```python
from build123d import *

# Parameters (mm, degrees)
SKETCH1_W           = 29
SKETCH1_H           = 39
BOSS_EXTRUDE1_DEPTH = 40
SKETCH2_R           = 10.1
BOSS_EXTRUDE2_DEPTH = 33
SKETCH3_R           = 20
BOSS_EXTRUDE3_DEPTH = 2.5
FILLET1_R           = 5


with BuildPart() as part:
    # Sketch1 → Boss-Extrude1 (new body)
    with BuildSketch(Plane(origin=(0, 0, 0), x_dir=(1, 0, 0), z_dir=(0, 1, 0))):
        Rectangle(SKETCH1_W, SKETCH1_H)
    extrude(amount=BOSS_EXTRUDE1_DEPTH)

    # Sketch2 → Boss-Extrude2 (add)
    with BuildSketch(Plane(origin=(0, 40, 0), x_dir=(1, 0, 0), z_dir=(0, 1, 0))):
        with Locations(Location((0, 0, 0), (0, 0, 270))):
            Circle(SKETCH2_R)
    extrude(amount=BOSS_EXTRUDE2_DEPTH)

    # Sketch3 → Boss-Extrude3 (add)
    with BuildSketch(Plane(origin=(0, 73, 0), x_dir=(1, 0, 0), z_dir=(0, 1, 0))):
        with Locations(Location((0, 0, 0), (0, 0, 270))):
            Circle(SKETCH3_R)
    extrude(amount=-BOSS_EXTRUDE3_DEPTH)

    # Fillet1
    # the kernel refuses this fillet: 5 mm, written as the material it takes off along each edge
    with BuildSketch(Plane(origin=(0, 73, 0), x_dir=(0, 0, 1), z_dir=(-1, 0, 0))) as fillet1_piece_1:
        with BuildLine():
            CenterArc((15.669872981, -5), FILLET1_R, 30, 60)
            Line((15.669872981, 0), (15.669872981, 0.1))
            Line((15.669872981, 0.1), (20, 0.1))
            Line((20, 0.1), (20.1, 0))
            ThreePointArc((20.1, 0), (20.1, -1.25), (20.08660254, -2.45))
            Line((20.08660254, -2.45), (20, -2.5))
        make_face()
    revolve(axis=Axis((0, 73, 0), (0, 1, 0)), mode=Mode.SUBTRACT)


solid = part.part
```
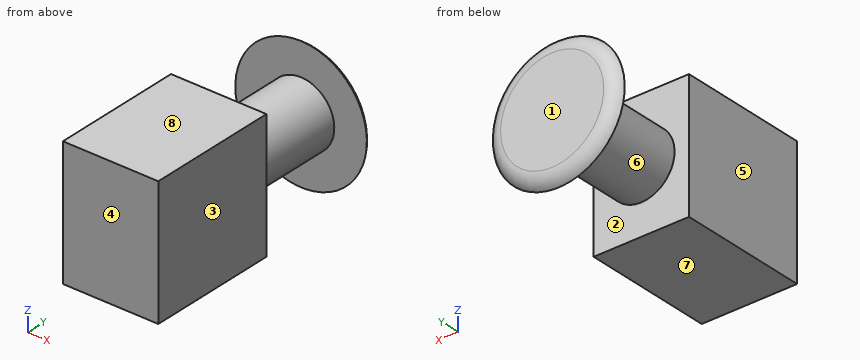
Can you work these out from the model? Positions are in its coordinate system, mm. Face numbers are marked on the shaded views. A direction names the side the tool comes from. Coordinates: 2 decimals unless noted, no trailing zeros. Loops run counter-clockwise (first coordinate to the right, second up) from the corner with the lowest first, then second, coordinate; pieces in that order, holes last. Notation, with made-up numbers: (-18, 67.25) - (16, 67.25) arc R19 cw to (16, 79.25) - close; hole circle Ø3 at (-29.5, 76.5). An arc over 180 degrees is marked (long way). Use a Markdown table: item, result.
Item 1: For the marked faces 5, 6, 7 and 8, which set-ups out of +Z, -Z, +X, -X, +Y, -Y let a thin tool reach every point of the face, with its end or its side?
Numbers:
| item | result |
|---|---|
| face 5 | +Z, -Z, -X, -Y |
| face 6 | none |
| face 7 | -Z, +X, -X, -Y |
| face 8 | +Z, +X, -X, -Y |
Item 2: I want a section at D-D on y = 59.5. Please give me the cut outline in (x, z).
Numbers:
| item | result |
|---|---|
| outline | circle Ø20.2 at (0, 0) |
Item 3: I want a section at A-A on z = 0. Please give me the cut outline in (x, y).
Numbers:
| item | result |
|---|---|
| outline | (-20, 70.5) - (-10.1, 70.5) - (-10.1, 40) - (-14.5, 40) - (-14.5, 0) - (14.5, 0) - (14.5, 40) - (10.1, 40) - (10.1, 70.5) - (20, 70.5) arc R5 ccw to (15.67, 73) - (-15.67, 73) arc R5 ccw to start |
Item 4: I want a section at B-B on x = 0. Please give me the cut outline in (y, z).
Numbers:
| item | result |
|---|---|
| outline | (0, -19.5) - (40, -19.5) - (40, -10.1) - (70.5, -10.1) - (70.5, -20) arc R5 ccw to (73, -15.67) - (73, 15.67) arc R5 ccw to (70.5, 20) - (70.5, 10.1) - (40, 10.1) - (40, 19.5) - (0, 19.5) - close |
Item 5: If I drill on probe 1 along X at (y, z) = (13.5, 4); probe 2 along Z at (x, y) = (5, 39.5); probe 3 along Y at (x, z) = (-13.5, 16.5), over which ranges is the centre line in solid material (lowest first)? Write a range as from..to.
Numbers:
| item | result |
|---|---|
| probe 1 | x = -14.5..14.5 |
| probe 2 | z = -19.5..19.5 |
| probe 3 | y = 0..40 |
Item 6: Will these pins go through, and if not, where does the flat tip stop? pin 1 (12 mm diameter, centred on y = 51, z = 5.5, fed in from +X); pin 2 (23 mm diameter, centred on x = -3.5, y = 27.5, fed in from -Z); pin 3 (11.5 mm diameter, centred on y = 23, z = 6.5, fed in from +X); pin 4 (4 mm diameter, centred on x = -7.5, z = 7, fed in from -Y).
Numbers:
| item | result |
|---|---|
| pin 1 | stops at x = 10.1 |
| pin 2 | stops at z = -19.5 |
| pin 3 | stops at x = 14.5 |
| pin 4 | stops at y = 0 |
Item 7: We'd pull the mould along Y, two halves only. Please class the marked faces 1, 2, 3 and 4: released by +Y, released by -Y, zero draft, split by the parting line, or undercut.
Numbers:
| item | result |
|---|---|
| face 1 | released by +Y |
| face 2 | undercut |
| face 3 | zero draft |
| face 4 | released by -Y |
Item 8: I want a section at C-C on y = 13. Please give me the cut outline in (x, z), and give its area (3 significant figures).
Numbers:
| item | result |
|---|---|
| outline | (-14.5, -19.5) - (14.5, -19.5) - (14.5, 19.5) - (-14.5, 19.5) - close |
| area | 1,130 mm2 |
